from build123d import *

# Parameters (mm, degrees)
P_IDAT_VYSUNUT_M2_DEPTH     = 16.5
SKICA2_W                    = 46
SKICA2_H                    = 170.5
SKICA2_W_2                  = 37
SKICA2_H_2                  = 161.5
P_IDAT_VYSUNUT_M4_DEPTH     = 2
SKICA3_W                    = 46
SKICA3_H                    = 170.5
SKICA3_W_2                  = 37
SKICA3_H_2                  = 33.5
P_IDAT_VYSUNUT_M5_DEPTH     = 3
SKICA4_W                    = 37
SKICA4_H                    = 33.5
P_IDAT_VYSUNUT_M6_DEPTH     = 2
SKICA9_W                    = 46
SKICA9_H                    = 170.5
SKICA9_W_2                  = 37
SKICA9_H_2                  = 161.5
P_IDAT_VYSUNUT_M9_DEPTH     = 2
SKICA10_R                   = 1.75
D_RY_NA_Z_PUSTN_MATKY_DEPTH = 5
ZAOBLIT1_R                  = 2.5
SKICA11_R                   = 5.75
KONEKTORY_DEPTH             = 4.5
DR_KA_K_TER_U_DEPTH         = 120


with BuildPart() as part:
    # Skica1 → Přidat vysunutím2 (new body)
    with BuildSketch(Plane.XY):
        Polygon((40, 157.5), (-6, 157.5), (-6, 0), (-6, -13), (40, -13), (40, 0), align=None)
        Polygon((-1.5, 0), (-1.5, 153), (35.5, 153), (35.5, 0), (35.5, -8.5), (-1.5, -8.5), align=None, mode=Mode.SUBTRACT)
    extrude(amount=-P_IDAT_VYSUNUT_M2_DEPTH)

    # Skica2 → Přidat vysunutím4 (add)
    with BuildSketch(Plane.XY):
        with Locations((17, 72.25)):
            Rectangle(SKICA2_W, SKICA2_H)
        with Locations((17, 72.25)):
            Rectangle(SKICA2_W_2, SKICA2_H_2, mode=Mode.SUBTRACT)
    extrude(amount=P_IDAT_VYSUNUT_M4_DEPTH)

    # Skica3 → Přidat vysunutím5 (add)
    with BuildSketch(Plane.XY.offset(2)):
        with Locations((17, 72.25)):
            Rectangle(SKICA3_W, SKICA3_H)
        with Locations((17, 136.25)):
            Rectangle(SKICA3_W_2, SKICA3_H_2, mode=Mode.SUBTRACT)
    extrude(amount=P_IDAT_VYSUNUT_M5_DEPTH)

    # Skica4 → Přidat vysunutím6 (add)
    with BuildSketch(Plane.XY.offset(5)):
        with Locations((17, 136.25)):
            Rectangle(SKICA4_W, SKICA4_H)
    extrude(amount=-P_IDAT_VYSUNUT_M6_DEPTH)

    # Skica9 → Přidat vysunutím9 (add)
    with BuildSketch(Plane(origin=(0, 0, -16.5), x_dir=(-1, 0, 0), z_dir=(0, 0, -1))):
        with Locations((-17, 72.25)):
            Rectangle(SKICA9_W, SKICA9_H)
        with Locations((-17, 72.25)):
            Rectangle(SKICA9_W_2, SKICA9_H_2, mode=Mode.SUBTRACT)
    extrude(amount=P_IDAT_VYSUNUT_M9_DEPTH)

    # Skica10 → Díry na zápustný matky (cut)
    with BuildSketch(Plane(origin=(0, 0, -18.5), x_dir=(-1, 0, 0), z_dir=(0, 0, -1))):
        with Locations((3.5, -10.5)):
            Circle(SKICA10_R)
        with Locations((-37.5, -10.5)):
            Circle(SKICA10_R)
        with Locations((-37.5, 30.5)):
            Circle(SKICA10_R)
        with Locations((-37.5, 71.5)):
            Circle(SKICA10_R)
        with Locations((-37.5, 112.5)):
            Circle(SKICA10_R)
        with Locations((-37.5, 153.5)):
            Circle(SKICA10_R)
        with Locations((3.5, 30.5)):
            Circle(SKICA10_R)
        with Locations((3.5, 71.5)):
            Circle(SKICA10_R)
        with Locations((3.5, 112.5)):
            Circle(SKICA10_R)
        with Locations((3.5, 153.5)):
            Circle(SKICA10_R)
    extrude(amount=-D_RY_NA_Z_PUSTN_MATKY_DEPTH, mode=Mode.SUBTRACT)

    # Zaoblit1
    zaoblit1_edges = [part.edges().sort_by_distance(p)[0] for p in [
        (-1.5, 153, -7.75),
        (35.5, 153, -7.75),
        (35.5, -8.5, -8.25),
        (-1.5, -8.5, -8.25),
    ]]
    fillet(zaoblit1_edges, radius=ZAOBLIT1_R)

    # Skica11 → konektory (cut)
    with BuildSketch(Plane.XZ.offset(13)):
        with Locations(Location((27, -6.5, 0), (0, 0, 270))):
            Circle(SKICA11_R)
        with Locations(Location((7, -6.5, 0), (0, 0, 180))):
            Circle(SKICA11_R)
    extrude(amount=-KONEKTORY_DEPTH, mode=Mode.SUBTRACT)

    # Skica13 → Drážka k terču (cut)
    with BuildSketch(Plane.XZ.offset(13)):
        Polygon((31.5, 3), (25.5, 3), (27, 5), (30, 5), align=None)
        Polygon((7, 5), (4, 5), (2.5, 3), (8.5, 3), align=None)
    extrude(amount=-DR_KA_K_TER_U_DEPTH, mode=Mode.SUBTRACT)


solid = part.part
Check sheet for the modelled part. Datum: model origin and axes. Units: mm. A direction names the side the tool comes from. Give positions to 0.01 mm unless a question says otherwise; leave off trailing zeros. Write each loop counter-clockwise with the first axis right and the second up, starting at its lowest first coordinate (ties: lowest second). Pieces come first, ordered by that corner, then holes. Notation, with made-up numbers: (45, 34.5) -> (84, 34.5) arc R25 ccw to (84, 71.5) -> close; hole circle Ø11 at (88, 20.5). An arc over 180 degrees is marked (long way). Use one line per item in the form item = value. Start each with the question number.
1. Section check D-D (y = -10.5). Record the cut outline in (x, z).
2. Access from +Z, -Z, +X, -X, +Y, -Y to the whole of each face (thin tool, end or side, straight path). Record for faces 4 (the cylindrical face through (1.516, -10.782, -8.227)), 5 (the cylindrical face through (36.6, 155, -16)), 6 (the flat face through (17, 73, 5)).
3. Section check C-C (x = 17.5). Record the cut outline in (y, z).
4. Section check B-B (y = 14.5). Record the cut outline in (x, z), and give its area (4 significant figures).
5. Mould release check, pull along Z, two halves, no side actions. Record for faces 1 (the flat face through (29, 46, 3)), 2 (the flat face through (36, 73, -18.5)), 3 (the cylindrical face through (-3.272, 114.235, -16.035)): pulls with the +Z half, pulls with the -Z half, needs draft (parallel to the pull), parting line crosses it, or undercut.
6. Go/stop test with flat-tipped pins: P1, Ø5, axis at x = 15, y = 58.5, coming from the -Z side; P2, Ø1, axis at x = 37, y = -10.5, coming from the -Z side; P3, Ø1, axis at x = 27, z = 4, coming from the -Y side. Record where each tip stops, or that it passes through.
7. Thickness scan on line 1 along X through (y, z) = (153.5, -16.5); line 2 along X through (y, z) = (71.5, -17.35); line 3 along Y through (x, z) = (-3.5, -14.65). Record the ranges inside material, lowest first. Write a range as from..to.
8. Section check A-A (z = -6.5). Record the cut outline in (x, y), and give its area (3 significant figures).
Conclusion:
q1.outline = (-6, -18.5) -> (-5.25, -18.5) -> (-5.25, -13.5) -> (-1.75, -13.5) -> (-1.75, -18.5) -> (35.75, -18.5) -> (35.75, -13.5) -> (39.25, -13.5) -> (39.25, -18.5) -> (40, -18.5) -> (40, 5) -> (30, 5) -> (31.5, 3) -> (25.5, 3) -> (27, 5) -> (7, 5) -> (8.5, 3) -> (2.5, 3) -> (4, 5) -> (-6, 5) -> close; hole circle Ø11.5 at (7, -6.5); hole circle Ø11.5 at (27, -6.5)
q2.face_4 = -Y
q2.face_5 = -Z
q2.face_6 = +Z, +X, -X, +Y, -Y
q3.outline = (-13, -18.5) -> (-8.5, -18.5) -> (-8.5, 2) -> (119.5, 2) -> (119.5, 3) -> (153, 3) -> (153, -18.5) -> (157.5, -18.5) -> (157.5, 5) -> (-13, 5) -> close
q4.outline = (-6, -18.5) -> (-1.5, -18.5) -> (-1.5, 2) -> (35.5, 2) -> (35.5, -18.5) -> (40, -18.5) -> (40, 5) -> (30, 5) -> (31.5, 3) -> (25.5, 3) -> (27, 5) -> (7, 5) -> (8.5, 3) -> (2.5, 3) -> (4, 5) -> (-6, 5) -> close
q4.area = 304.5 mm²
q5.face_1 = undercut
q5.face_2 = pulls with the -Z half
q5.face_3 = needs draft
q6.P1 = 2
q6.P2 = -13.5
q6.P3 = 107
q7.line_1 = -6..-5.25, -1.75..35.75, 39.25..40
q7.line_2 = -6..-5.25, -1.75..-1.5, 35.5..35.75, 39.25..40
q7.line_3 = -13..-12.25, -8.75..28.75, 32.25..69.75, 73.25..110.75, 114.25..151.75, 155.25..157.5
q8.outline = (-6, -13) -> (1.25, -13) -> (1.25, -8.5) -> (1, -8.5) arc R2.5 cw to (-1.5, -6) -> (-1.5, 150.5) arc R2.5 cw to (1, 153) -> (33, 153) arc R2.5 cw to (35.5, 150.5) -> (35.5, -6) arc R2.5 cw to (33, -8.5) -> (32.75, -8.5) -> (32.75, -13) -> (40, -13) -> (40, 157.5) -> (-6, 157.5) -> close; (12.75, -13) -> (21.25, -13) -> (21.25, -8.5) -> (12.75, -8.5) -> close
q8.area = 1,770 mm²
